The model under review builds one solid part; all positions refer to its coordinate system, in mm. Face numbers are marked on the shaded views. A direction names the side the tool comes from. Coordinates: 2 decimals unless noted, no trailing zeros. Write each loop counter-clockwise with the first axis right and the second up, starting at its lowest first coordinate (ties: lowest second). Pieces come first, ordered by that corner, then holes. Notation, with made-up numbers: (75.5, 51.25) -> (94.5, 51.25) arc R11 cw to (94.5, 68.25) -> close; hole circle Ø1 at (-21, 84.25). An arc over 180 degrees is marked (long way). Put each result on its own line as item: value. Start each with the question number.
from build123d import *

# Parameters (mm, degrees)
F1_DEPTH = 45
F2_T     = -2
F4_DEPTH = 3


with BuildPart() as f1:
    # F0 (on Top) → F1 (new body)
    with BuildSketch(Plane.XY):
        with BuildLine():
            ThreePointArc((0, 3), (0.87868, 0.87868), (3, 0))
            Line((3, 0), (29, 0))
            ThreePointArc((29, 0), (31.12132, 0.87868), (32, 3))
            Line((32, 3), (32, 49))
            ThreePointArc((32, 49), (31.12132, 51.12132), (29, 52))
            Line((29, 52), (3, 52))
            ThreePointArc((3, 52), (0.87868, 51.12132), (0, 49))
            Line((0, 49), (0, 3))
        make_face()
    extrude(amount=F1_DEPTH)

    # F2
    f2_openings = [f1.faces().sort_by_distance(p)[0] for p in [
        (16, 26, 45),
    ]]
    offset(amount=F2_T, openings=f2_openings)

    # F3 (on face) → F4 (join)
    with BuildSketch(Plane.XY.offset(45)):
        with BuildLine():
            Line((29, 50.8), (3, 50.8))
            ThreePointArc((3, 50.8), (1.727208, 50.272792), (1.2, 49))
            Line((1.2, 49), (1.2, 3))
            ThreePointArc((1.2, 3), (1.727208, 1.727208), (3, 1.2))
            Line((3, 1.2), (29, 1.2))
            ThreePointArc((29, 1.2), (30.272792, 1.727208), (30.8, 3))
            Line((30.8, 3), (30.8, 49))
            ThreePointArc((30.8, 49), (30.272792, 50.272792), (29, 50.8))
        make_face()
        with BuildLine():
            Line((29, 2), (3, 2))
            ThreePointArc((3, 2), (2.292893, 2.292893), (2, 3))
            Line((2, 3), (2, 49))
            ThreePointArc((2, 49), (2.292893, 49.707107), (3, 50))
            Line((3, 50), (29, 50))
            ThreePointArc((29, 50), (29.707107, 49.707107), (30, 49))
            Line((30, 49), (30, 3))
            ThreePointArc((30, 3), (29.707107, 2.292893), (29, 2))
        make_face(mode=Mode.SUBTRACT)
    extrude(amount=F4_DEPTH)


solid = f1.part
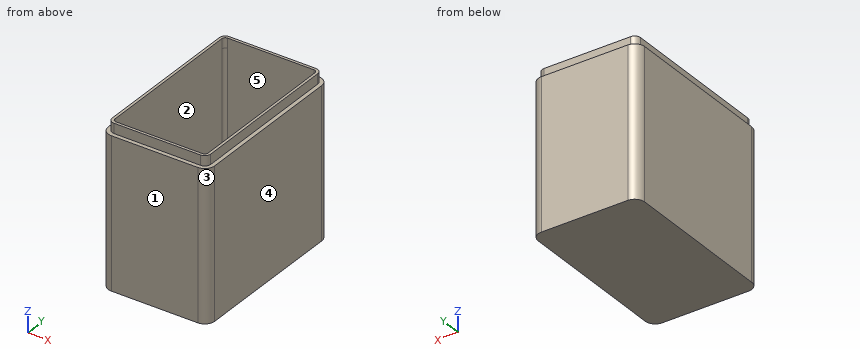
1. Tool access review of the marked faces 4 and 5: name each direction out of +Z, -Z, +X, -X, +Y, -Y from which nothing blocks a thin tool from reaching the whole face with its end or side.
2. Consider section B-B on y = 36. State the section outline as (x, z) points.
3. The part is to be moulded in two halves that separate along X. For the marked faces 1, 2 and 3, say which applies: released by +X, released by -X, zero draft, split by the parting line, or undercut.
4. Wall thickness on line 1 (X direction, y = 39, z = 26); line 2 (Y direction, x = 8.5, z = 9); line 3 (Y direction, x = 8, z = 46): over which ranges is each line inside the solid? List them lowest first. Write a range as from..to.
5. Consider section A-A on z = 30. State the section outline as (x, y) points.
6. Insertion check: P1, Ø8.5, axis at x = 20.5, y = 17.5, coming from the +Z side; P2, Ø0.9, axis at x = 18, z = 47, coming from the -Y side; P3, Ø0.9, axis at x = 15.5, z = 47, coming from the +Y side. Each pin has a flat end and moves straight along its axis. Give the tip position at first contact, or say it passes through.
7. Consider section C-C on x = 26. State the section outline as (y, z) points, then the cut area to 3 significant figures.
Output values:
1. face 4: +Z, -Z, +X, +Y, -Y
1. face 5: +Z
2. outline: (0, 0) -> (32, 0) -> (32, 45) -> (30.8, 45) -> (30.8, 48) -> (30, 48) -> (30, 2) -> (2, 2) -> (2, 48) -> (1.2, 48) -> (1.2, 45) -> (0, 45) -> close
3. face 1: zero draft
3. face 2: undercut
3. face 3: released by +X
4. line 1: x = 0..2, 30..32
4. line 2: y = 0..2, 50..52
4. line 3: y = 1.2..2, 50..50.8
5. outline: (0, 3) arc R3 ccw to (3, 0) -> (29, 0) arc R3 ccw to (32, 3) -> (32, 49) arc R3 ccw to (29, 52) -> (3, 52) arc R3 ccw to (0, 49) -> close; hole (2, 3) arc R1 ccw to (3, 2) -> (29, 2) arc R1 ccw to (30, 3) -> (30, 49) arc R1 ccw to (29, 50) -> (3, 50) arc R1 ccw to (2, 49) -> close
6. P1: stops at z = 2
6. P2: stops at y = 1.2
6. P3: stops at y = 50.8
7. outline: (0, 0) -> (52, 0) -> (52, 45) -> (50.8, 45) -> (50.8, 48) -> (50, 48) -> (50, 2) -> (2, 2) -> (2, 48) -> (1.2, 48) -> (1.2, 45) -> (0, 45) -> close
7. area: 281 mm^2
